from build123d import *

# Parameters (mm, degrees)
IZIM1_R                     = 10
IZIM1_R_2                   = 5
Y_KSEKLIK_EKSTR_ZYON1_DEPTH = 5
PAH1_SIZE                   = 5
IZIM2_R                     = 1
KANCA_DELIKLERI_DEPTH       = 204.010978335


with BuildPart() as part:
    # Çizim1 → Yükseklik-Ekstrüzyon1 (new body)
    # profile 1 of 2: a face of its own
    with BuildSketch(Plane(origin=(0, 0, 0), x_dir=(1, 0, 0), z_dir=(0, 1, 0))):
        Circle(IZIM1_R)
        with Locations(Location((0, 0, 0), (0, 0, 270))):
            Circle(IZIM1_R_2, mode=Mode.SUBTRACT)
    # profile 2 of 2: a face of its own
    with BuildSketch(Plane(origin=(0, 0, 0), x_dir=(1, 0, 0), z_dir=(0, 1, 0))):
        with BuildLine():
            ThreePointArc((2.57e-07, -10), (96.592582662, 64.118095614), (50, 176.602540378))
            ThreePointArc((50, 176.602540378), (50.573117628, 85.626381928), (0, 10))
            ThreePointArc((0, 10), (7.071067812, 7.071067812), (10, 0))
            ThreePointArc((10, 0), (7.071067903, -7.071067721), (2.57e-07, -10))
        make_face()
    extrude(amount=Y_KSEKLIK_EKSTR_ZYON1_DEPTH)

    # Pah1
    pah1_edges = [part.edges().sort_by_distance(p)[0] for p in [
        (50.573117628, 5, -85.626381928),
    ]]
    chamfer(pah1_edges, length=PAH1_SIZE - 0.0001)  # a hair under: the kernel refuses the full size

    # Çizim2 → kanca delikleri (cut, through all)
    with BuildSketch(Plane(origin=(0, 5, 0), x_dir=(1, 0, 0), z_dir=(0, 1, 0))):
        with Locations(Location((69.348523033, 154.929056309, 0), (0, 0, 270))):
            Circle(IZIM2_R)
        with Locations(Location((85.505252147, 131.398693884, 0), (0, 0, 270))):
            Circle(IZIM2_R)
        with Locations(Location((93.943127486, 104.131128696, 0), (0, 0, 270))):
            Circle(IZIM2_R)
        with Locations(Location((93.900432964, 75.587897823, 0), (0, 0, 270))):
            Circle(IZIM2_R)
        with Locations(Location((85.381022764, 48.345697079, 0), (0, 0, 270))):
            Circle(IZIM2_R)
        with Locations(Location((69.153973403, 24.863773807, 0), (0, 0, 270))):
            Circle(IZIM2_R)
        with Locations(Location((46.684156547, 7.261922143, 0), (0, 0, 270))):
            Circle(IZIM2_R)
        with Locations(Location((20, -2.870878105, 0), (0, 0, 270))):
            Circle(IZIM2_R)
    extrude(amount=-KANCA_DELIKLERI_DEPTH, mode=Mode.SUBTRACT)


solid = part.part
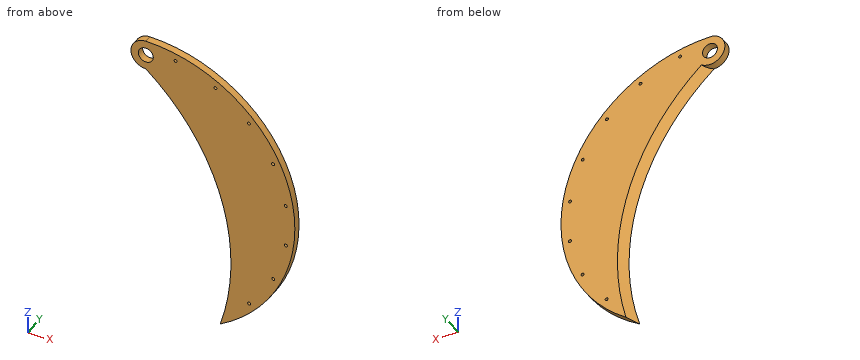
Model file for the job. Use its own axes, mm. Give positions to 0.01 mm unless a question says otherwise; leave off trailing zeros. Order: outer loops, then holes, each group sorted by start corner. A loop starts at its lowest first (then second) coordinate and runs counter-clockwise, first axis right, second up. Notation, with made-up numbers: (-30, 88.25) -> (8, 88.25) arc R12 ccw to (8, 95.25) -> close; hole circle Ø6 at (12.5, 5). An arc over 180 degrees is marked (long way). Use CSV: the item, a comma, the result in double quotes.
1. Drop flat-ended pins along their axis: pin 1 (3 mm diameter, centred on x = 14.5, z = -27.5, fed in from -Y); pin 2 (1.5 mm diameter, centred on y = 2, z = -137.5, fed in from +X). Give the stop position or say it passes through.
Outcome:
pin 1,"through"
pin 2,"x = 88.4"
2. Band-saw the part on A-A, the plane y = 1.45. Count the separate pieces of the cut face and the enclosed holes in it, then the cut area to 3 significant figures.
Outcome:
separate pieces,"1"
enclosed holes,"9"
area,"7,720 mm²"
3. Drill centre lines: line 1 along Z through (x, y) = (69, 1.7); line 2 along X through (y, z) = (1.45, 0); line 3 along X through (y, z) = (2.85, -55). Where is each one in solid material? Low to high. Write a range as from..to.
Outcome:
line 1,"-162.38..-155.87, -153.99..-25.85, -23.88..-17.62"
line 2,"-10..-5, 5..43.59"
line 3,"40.91..93.67"
4. Band-saw the part on B-B, the plane z = 0. Give the cut face in (x, y), then the cut area to 3 significant figures.
Outcome:
outline,"(-10, 0) -> (-5, 0) -> (-5, 5) -> (-10, 5) -> close; (5, 0) -> (43.59, 0) -> (43.59, 5) -> (5, 5) -> close"
area,"218 mm²"
